Here's how the part is built. I have some questions about the finished solid (model axes, mm). Round coordinates to 2 decimals unless told otherwise and drop trailing zeros. Order: outer loops, then holes, each group sorted by start corner. A loop starts at its lowest first (then second) coordinate and runs counter-clockwise, first axis right, second up.
```python
from build123d import *

# Parameters (mm, degrees)
SKETCH1_R           = 23.57
SKETCH1_R_2         = 2.5
BOSS_EXTRUDE1_DEPTH = 5
SKETCH2_W           = 65
SKETCH2_H           = 3
CUT_EXTRUDE1_DEPTH  = 70


with BuildPart() as part:
    # Sketch1 → Boss-Extrude1 (new body)
    with BuildSketch(Plane.XY):
        with BuildLine():
            Line((-16.5, -28), (16.5, -28))
            ThreePointArc((16.5, -28), (0, 32.5), (-16.5, -28))
        make_face()
        Circle(SKETCH1_R, mode=Mode.SUBTRACT)
        with Locations((24.283327614, -14.06)):
            Circle(SKETCH1_R_2, mode=Mode.SUBTRACT)
        with Locations((24.32947184, 13.98)):
            Circle(SKETCH1_R_2, mode=Mode.SUBTRACT)
        with Locations((0, 28.358420848)):
            Circle(SKETCH1_R_2, mode=Mode.SUBTRACT)
        with Locations((-24.32947184, 13.98)):
            Circle(SKETCH1_R_2, mode=Mode.SUBTRACT)
        with Locations((-24.283327614, -14.06)):
            Circle(SKETCH1_R_2, mode=Mode.SUBTRACT)
    extrude(amount=BOSS_EXTRUDE1_DEPTH)

    # Sketch2 → Cut-Extrude1 (cut)
    with BuildSketch(Plane(origin=(0, -28, 0), x_dir=(-1, 0, 0), z_dir=(0, -1, 0))):
        with Locations((0, -1.5)):
            Rectangle(SKETCH2_W, SKETCH2_H)
    extrude(amount=-CUT_EXTRUDE1_DEPTH, mode=Mode.SUBTRACT)


solid = part.part
```
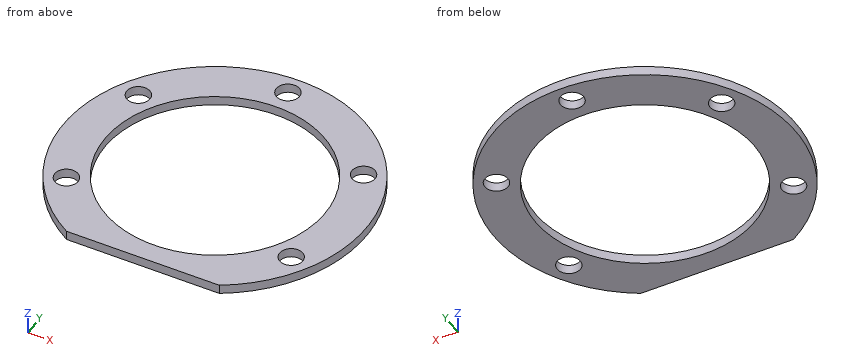
1. If we section it at D-D, the plane x = 6.5: Write out the boundary of the cut face in (y, z), and give its area (3 significant figures).
Evaluation:
outline: (-28, 3) - (-22.66, 3) - (-22.66, 5) - (-28, 5) - close; (22.66, 3) - (31.84, 3) - (31.84, 5) - (22.66, 5) - close
area: 29.1 mm2
2. I need wall thicknesses on probe 1 along Y at (x, z) = (0, 3.95); probe 2 along X at (y, z) = (-14.06, 4.35); probe 3 along Y at (x, z) = (-24.5, 3.3). Which ranges of each line are inside material? Lowest first, please.
Evaluation:
probe 1: y = -28 to -23.57, 23.57 to 25.86, 30.86 to 32.5
probe 2: x = -29.3 to -26.78, -21.78 to -18.92, 18.92 to 21.78, 26.78 to 29.3
probe 3: y = -21.35 to -16.55, -11.57 to 11.49, 16.47 to 21.35
3. If we section it at B-B, the plane x = 0: Write out the boundary of the cut face in (y, z), and give its area (3 significant figures).
Evaluation:
outline: (-28, 3) - (-23.57, 3) - (-23.57, 5) - (-28, 5) - close; (23.57, 3) - (25.86, 3) - (25.86, 5) - (23.57, 5) - close; (30.86, 3) - (32.5, 3) - (32.5, 5) - (30.86, 5) - close
area: 16.7 mm2
4. If we section it at A-A, the plane y = 0: Write out the boundary of the cut face in (x, z).
Evaluation:
outline: (-32.5, 3) - (-23.57, 3) - (-23.57, 5) - (-32.5, 5) - close; (23.57, 3) - (32.5, 3) - (32.5, 5) - (23.57, 5) - close
5. I'm going to push flat-ended pins straight in: P1, Ø4, axis at x = 24.33, y = 13.98, coming from the +Z side; P2, Ø1, axis at y = 16, z = 4.5, coming from the +X side. Where does each tip first touch, or does it pass through?
Evaluation:
P1: passes through
P2: stops at x = 28.57
6. If we section it at C-C, the plane y = -14.06: Write out the boundary of the cut face in (x, z), and give its area (3 significant figures).
Evaluation:
outline: (-29.3, 3) - (-26.78, 3) - (-26.78, 5) - (-29.3, 5) - close; (-21.78, 3) - (-18.92, 3) - (-18.92, 5) - (-21.78, 5) - close; (18.92, 3) - (21.78, 3) - (21.78, 5) - (18.92, 5) - close; (26.78, 3) - (29.3, 3) - (29.3, 5) - (26.78, 5) - close
area: 21.5 mm2
